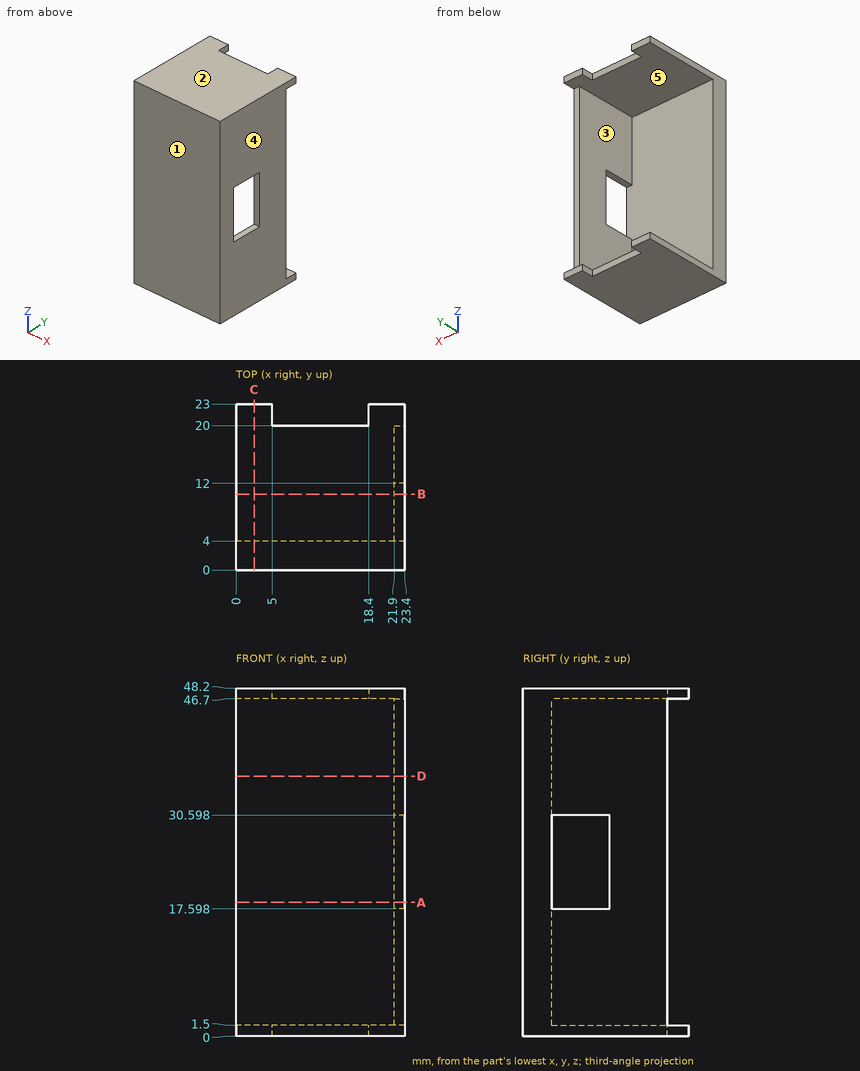
Design review of the part shown in the three views and the two pictorial views. Dimensions are in mm from the part's minimum x, y and z. A direction names the side the tool comes from. Round coordinates to 2 decimals unless told otherwise and drop trailing zeros. Order: outer loops, then holes, each group sorted by start corner. A loop starts at its lowest first (then second) coordinate and runs counter-clockwise, first axis right, second up. Notation, with made-up numbers: (-38.75, 27.25) -> (16.25, 27.25) arc R20 ccw to (16.25, 31.25) -> close; hole circle Ø10 at (8.25, -7). An arc over 180 degrees is marked (long way). Write item = value, one per line. Start each with the question number.
1) Tool access review of the marked faces 4 and 5: name each direction out of +Z, -Z, +X, -X, +Y, -Y from which nothing blocks a thin tool from reaching the whole face with its end or side.
2) Insertion check: pin 1 (5 mm diameter, centred on x = 17, z = 21, fed in from +Y); pin 2 (5 mm diameter, centred on y = 14.5, z = 13.5, fed in from -X); pin 3 (1.6 mm diameter, centred on x = 23, z = 17, fed in from +Y). Each pin has a flat end and moves straight along its axis. Give the tip position at first contact, or say it passes through.
3) Take a section at C-C on x = 2.5. State the section outline as (y, z) points, plus the area to 3 significant figures.
4) Take a section at B-B on y = 10.5. State the section outline as (x, z) points.
5) Take a section at D-D on z = 36. State the section outline as (x, y) points, plus the area to 3 significant figures.
6) To check wall thickness, follow line 1 (Z direction, x = 7, y = 8.25); line 2 (X direction, y = 15.75, z = 12); line 3 (Y direction, x = 21.5, z = 20). State the ranges of each line that lie inside material, in increasing order. Write a range as from..to.
7) Take a section at A-A on z = 18.5. State the section outline as (x, y) points.
8) The part is to be moulded in two halves that separate along Z. For the marked faces 1, 2 and 3, say which applies: +Z half, -Z half, draft (parallel to the pull), parting line (faces both ways), or undercut.
Verdict:
q1.face_4 = +Z, -Z, +X, +Y, -Y
q1.face_5 = -X, +Y
q2.pin_1 = 4
q2.pin_2 = 21.9
q2.pin_3 = 20
q3.outline = (0, 0) -> (23, 0) -> (23, 1.5) -> (4, 1.5) -> (4, 46.7) -> (23, 46.7) -> (23, 48.2) -> (0, 48.2) -> close
q3.area = 250 mm2
q4.outline = (0, 0) -> (23.4, 0) -> (23.4, 17.6) -> (21.9, 17.6) -> (21.9, 1.5) -> (0, 1.5) -> close; (0, 46.7) -> (21.9, 46.7) -> (21.9, 30.6) -> (23.4, 30.6) -> (23.4, 48.2) -> (0, 48.2) -> close
q5.outline = (0, 0) -> (23.4, 0) -> (23.4, 20) -> (21.9, 20) -> (21.9, 4) -> (0, 4) -> close
q5.area = 118 mm2
q6.line_1 = 0..1.5, 46.7..48.2
q6.line_2 = 21.9..23.4
q6.line_3 = 0..4
q7.outline = (0, 0) -> (23.4, 0) -> (23.4, 4) -> (0, 4) -> close; (21.9, 12) -> (23.4, 12) -> (23.4, 20) -> (21.9, 20) -> close
q8.face_1 = draft
q8.face_2 = +Z half
q8.face_3 = undercut
